Autodesk Inventor part; units mm, degrees
ref_plane "YZ Plane" through (0, 0, 0) normal (1, 0, 0) x (0, 1, 0)
ref_plane "XZ Plane" through (0, 0, 0) normal (0, 1, 0) x (-1, 0, 0)
ref_plane "XY Plane" through (0, 0, 0) normal (0, 0, 1) x (1, 0, 0)
sketch "Sketch1" plane through (0, 0, 0) normal (0, 1, 0) x (-1, 0, 0)
  line L0 (0, -53.34) -> (0, 53.34)
  line L1 (-24.5, 0) -> (24.5, 0)
  line L2 (24.5, 0) -> (-24.5, 0)
  line L3 (0, -53.34) -> (0, 53.34)
  line L4 (-17.5, 38.1) -> (-17.5, -38.1)
  line L5 (-17.5, -38.1) -> (17.5, -38.1)
  line L6 (17.5, -38.1) -> (17.5, 38.1)
  line L7 (17.5, 38.1) -> (-17.5, 38.1)
  line L8 (-17.5, -38.1) -> (17.5, 38.1) construction
  point P0 (0, 0)
  dimension "d1" = 76.2
  dimension "d2" = 35
extrude "Extrusion1" add sketch "Sketch1" along normal mid plane 20
sketch "Sketch2" plane through (0, 10, 0) normal (0, 1, 0) x (1, 0, 0)
  point P0 (0, 0)
  point P1 (0, 0)
hole "Hole1" at (0, 10, 0) direction (0, -1, 0) diameter 28.575 end through all counterbore diameter 31.13 counterbore depth 1.6
fillet "Fillet1" radius 3.175 4 edges at (17.5, 0, 38.1) (17.5, 0, -38.1) (-17.5, 0, 38.1) (-17.5, 0, -38.1)
sketch "Sketch3" plane through (-17.5, -10, -34.925) normal (-1, 0, 0) x (0, 0, 1)
  line L0 (0, 0) -> (0, 20)
  line L1 (69.85, 0) -> (0, 0)
  line L2 (69.85, 20) -> (69.85, 0)
  line L3 (0, 20) -> (69.85, 20)
  line L4 (0, 20) -> (0, 0)
  line L5 (0, 0) -> (69.85, 0)
  line L6 (69.85, 0) -> (69.85, 20)
  line L7 (69.85, 20) -> (0, 20)
  line L8 (0, 20) -> (0, 0)
  line L9 (19.36, 20) -> (50.49, 20)
  line L10 (34.925, 20) -> (34.925, 0)
  line L11 (0, 10) -> (69.85, 10)
  line L12 (69.85, 0) -> (69.85, 20)
  point P0 (34.925, 10)
  point P1 (9.525, 10)
  point P2 (60.325, 10)
  dimension "d19" = 25.4
  dimension "d20" = 25.4
hole "Hole2" at (-17.5, 0, -25.4) at (-17.5, 0, 25.4) direction (1, 0, 0) diameter 5.08 end through all counterbore diameter 8.255 counterbore depth 10.16
properties part number "BearingBlock30mm"
Geometry check sheet. Reference: the model listing, model coordinates, mm. A direction names the side the tool comes from. Round coordinates to 2 decimals unless told otherwise and drop trailing zeros. Order: outer loops, then holes, each group sorted by start corner. A loop starts at its lowest first (then second) coordinate and runs counter-clockwise, first axis right, second up. Notation, with made-up numbers: M -34,-28.5 L -5,-28.5 A4 cw -5,-21.5 Z; hole C -21,-5 d2. An arc over 180 degrees is marked long. Write each question's results on one line, items separated by ' | '. Start each with the question number.
1. Draft check along Y on faces 4 (the face through (-7.34, -0.1, -22.7)), 5 (the face through (16, 10, 1)), 6 (the face through (0, 0, -38.1)). Enter one of: pulls with the +Y half, pulls with the -Y half, needs draft (parallel to the pull), parting line crosses it, or undercut.
2. Set-up check for faces 1 (the face through (15.195, 9.189, -3.374)), 2 (the face through (16.59, -0.14, 37.15)), 3 (the face through (-12.349, -0.181, -29.524)): record each of +Z, -Z, +X, -X, +Y, -Y from which the full face is reachable in a straight line by a thin tool's end or side.
3. Cross-section at B-B on x = 0. Record the boundary of the cut face in (y, z) (1 decimal).
4. Material ranges on L1, parallel to Y at x = 10.25, z = -25.4; L2, parallel to Z at x = -12.5, y = -2.25; L3, parallel to Z at x = -14.75, y = 0, recorded low to high. Write a range as from..to.
5. Cross-section at A-A on z = 0. Record the boundary of the cut face in (x, y) (1 decimal).
6. Cross-section at C-C on y = 0. Give the number of separate pieces and of enclosed holes in the cut face, plus the area to 3 significant figures.
7. Go/stop test with a flat-tipped pin: P1, Ø7.5, axis at y = 0, z = 25.4, coming from the -X side. Record where the tip stops, or that it passes through.
Resolved:
1) face 4: undercut | face 5: pulls with the +Y half | face 6: needs draft
2) face 1: +Y | face 2: +Z, +X, +Y, -Y | face 3: -X
3) outline: M -10,-38.1 L 10,-38.1 L 10,-15.6 L 8.4,-15.6 L 8.4,-14.3 L -10,-14.3 Z; M -10,14.3 L 8.4,14.3 L 8.4,15.6 L 10,15.6 L 10,38.1 L -10,38.1 Z; hole C 0,-25.4 d5.1; hole C 0,25.4 d5.1
4) L1: -10..-2.54, 2.54..10 | L2: -38.1..-28.86, -21.94..-6.92, 6.92..21.94, 28.86..38.1 | L3: -38.07..-29.53, -21.27..21.27, 29.53..38.07
5) outline: M -17.5,-10 L -14.3,-10 L -14.3,8.4 L -15.6,8.4 L -15.6,10 L -17.5,10 Z; M 14.3,-10 L 17.5,-10 L 17.5,10 L 15.6,10 L 15.6,8.4 L 14.3,8.4 Z
6) separate pieces: 3 | enclosed holes: 1 | area: 1,600 mm2
7) P1: x = -7.34
